For this review, take the finished solid that the model builds, in its own axes (mm). Face numbers are marked on the shaded views. Round coordinates to 2 decimals unless told otherwise and drop trailing zeros. Write each loop counter-clockwise with the first axis right and the second up, starting at its lowest first coordinate (ties: lowest second). Pieces come first, ordered by that corner, then holes. Notation, with made-up numbers: (-28, 29.25) -> (20, 29.25) arc R27 ccw to (20, 60.25) -> close; hole circle Ø7 at (31, 83). An arc over 180 degrees is marked (long way). Answer in a Markdown table with one row per item.
from build123d import *

# Parameters (mm, degrees)
BOSS_EXTRUDE1_DEPTH    = 2.6
BOSS_EXTRUDE2_START    = -2.6
BOSS_EXTRUDE2_DEPTH    = 69
BOSS_EXTRUDE3_START    = 3.2
BOSS_EXTRUDE3_DEPTH    = 2.6
FILL_START             = -63.4
FILL_PATTERN1_DEPTH    = 2.6
FILL_START_2           = -57.9
FILL_PATTERN1_2_DEPTH  = 2.6
FILL_START_3           = -52.4
FILL_PATTERN1_3_DEPTH  = 2.6
FILL_START_4           = -46.9
FILL_PATTERN1_4_DEPTH  = 2.6
FILL_START_5           = -41.4
FILL_PATTERN1_5_DEPTH  = 2.6
FILL_START_6           = -35.9
FILL_PATTERN1_6_DEPTH  = 2.6
FILL_START_7           = -30.4
FILL_PATTERN1_7_DEPTH  = 2.6
FILL_START_8           = -24.9
FILL_PATTERN1_8_DEPTH  = 2.6
FILL_START_9           = -19.4
FILL_PATTERN1_9_DEPTH  = 2.6
FILL_START_10          = -13.9
FILL_PATTERN1_10_DEPTH = 2.6
BOSS_EXTRUDE4_DEPTH    = 14
BOSS_EXTRUDE5_DEPTH    = 1.2
SKETCH6_W              = 9.5
SKETCH6_H              = 1.2
CUT_EXTRUDE1_DEPTH     = 3
CHAMFER1_START         = -1
CHAMFER1_DEPTH         = 3.165267299


with BuildPart() as part:
    # Sketch2 → Boss-Extrude1 (new body)
    with BuildSketch(Plane(origin=(0, 0, 0), x_dir=(0, 0, -1), z_dir=(1, 0, 0))):
        Polygon((0, 0), (0, 5.5), (7.5, 0), align=None)
    boss_extrude1 = extrude(amount=-BOSS_EXTRUDE1_DEPTH)

    # Sketch3 → Boss-Extrude2 (add)
    with BuildSketch(Plane.ZY.offset(2.6).offset(BOSS_EXTRUDE2_START)):
        Polygon((0, 0), (0, 4.879964159), (-6.65449658, 0), align=None)
    extrude(amount=BOSS_EXTRUDE2_DEPTH)

    # Sketch3<3> → Boss-Extrude3 (add)
    with BuildSketch(Plane.ZY.offset(2.6).offset(BOSS_EXTRUDE3_START)):
        Polygon((-6.65449658, 0), (0, 4.879964159), (0, 5.5), (-7.5, 0), align=None)
    extrude(amount=BOSS_EXTRUDE3_DEPTH)

    # Mirror1: Boss-Extrude1 across plane
    add(boss_extrude1.mirror(Plane(origin=(-34.5, 0, 0), x_dir=(0, 0, 1), z_dir=(1, 0, 0))))

    # Fill Pattern1: read off the stored shape, not the designer's step
    # Fill Pattern1 outline → Fill Pattern1 (add)
    with BuildSketch(Plane.YZ.offset(FILL_START)):
        Polygon((4.879964159, 0), (0, -6.65449658), (0, -7.5), (5.5, 0), align=None)
    extrude(amount=FILL_PATTERN1_DEPTH)

    # Fill Pattern1 2 outline → Fill Pattern1 2 (add)
    with BuildSketch(Plane.YZ.offset(FILL_START_2)):
        Polygon((4.879964159, 0), (0, -6.65449658), (0, -7.5), (5.5, 0), align=None)
    extrude(amount=FILL_PATTERN1_2_DEPTH)

    # Fill Pattern1 3 outline → Fill Pattern1 3 (add)
    with BuildSketch(Plane.YZ.offset(FILL_START_3)):
        Polygon((4.879964159, 0), (0, -6.65449658), (0, -7.5), (5.5, 0), align=None)
    extrude(amount=FILL_PATTERN1_3_DEPTH)

    # Fill Pattern1 4 outline → Fill Pattern1 4 (add)
    with BuildSketch(Plane.YZ.offset(FILL_START_4)):
        Polygon((4.879964159, 0), (0, -6.65449658), (0, -7.5), (5.5, 0), align=None)
    extrude(amount=FILL_PATTERN1_4_DEPTH)

    # Fill Pattern1 5 outline → Fill Pattern1 5 (add)
    with BuildSketch(Plane.YZ.offset(FILL_START_5)):
        Polygon((4.879964159, 0), (0, -6.65449658), (0, -7.5), (5.5, 0), align=None)
    extrude(amount=FILL_PATTERN1_5_DEPTH)

    # Fill Pattern1 6 outline → Fill Pattern1 6 (add)
    with BuildSketch(Plane.YZ.offset(FILL_START_6)):
        Polygon((4.879964159, 0), (0, -6.65449658), (0, -7.5), (5.5, 0), align=None)
    extrude(amount=FILL_PATTERN1_6_DEPTH)

    # Fill Pattern1 7 outline → Fill Pattern1 7 (add)
    with BuildSketch(Plane.YZ.offset(FILL_START_7)):
        Polygon((4.879964159, 0), (0, -6.65449658), (0, -7.5), (5.5, 0), align=None)
    extrude(amount=FILL_PATTERN1_7_DEPTH)

    # Fill Pattern1 8 outline → Fill Pattern1 8 (add)
    with BuildSketch(Plane.YZ.offset(FILL_START_8)):
        Polygon((4.879964159, 0), (0, -6.65449658), (0, -7.5), (5.5, 0), align=None)
    extrude(amount=FILL_PATTERN1_8_DEPTH)

    # Fill Pattern1 9 outline → Fill Pattern1 9 (add)
    with BuildSketch(Plane.YZ.offset(FILL_START_9)):
        Polygon((4.879964159, 0), (0, -6.65449658), (0, -7.5), (5.5, 0), align=None)
    extrude(amount=FILL_PATTERN1_9_DEPTH)

    # Fill Pattern1 10 outline → Fill Pattern1 10 (add)
    with BuildSketch(Plane.YZ.offset(FILL_START_10)):
        Polygon((4.879964159, 0), (0, -6.65449658), (0, -7.5), (5.5, 0), align=None)
    extrude(amount=FILL_PATTERN1_10_DEPTH)

    # Sketch4 → Boss-Extrude4 (add)
    with BuildSketch(Plane.ZY.offset(69)):
        with BuildLine():
            Line((0, 2.406191741), (0, 4.879964159))
            Line((0, 4.879964159), (-3.932237623, 1.996323235))
            ThreePointArc((-3.932237623, 1.996323235), (-1.977221876, 2.307779179), (0, 2.406191741))
        make_face()
        with BuildLine():
            Line((0, 4.879964159), (0, 5.5))
            Line((0, 5.5), (-5.225299515, 1.668113689))
            ThreePointArc((-5.225299515, 1.668113689), (-4.581760916, 1.844007543), (-3.932237623, 1.996323235))
            Line((-3.932237623, 1.996323235), (0, 4.879964159))
        make_face()
        with BuildLine():
            Line((-5.225299515, 1.668113689), (0, 5.5))
            Line((0, 5.5), (3.5, 5.5))
            Line((3.5, 5.5), (3.5, 8.5))
            Line((3.5, 8.5), (1.525445934, 8.5))
            Line((1.525445934, 8.5), (-9.5, 2.081639323))
            Line((-9.5, 2.081639323), (-9.5, -0.204677967))
            ThreePointArc((-9.5, -0.204677967), (-7.422606569, 0.868570996), (-5.225299515, 1.668113689))
        make_face()
    boss_extrude4 = extrude(amount=BOSS_EXTRUDE4_DEPTH)

    # Sketch5 → Boss-Extrude5 (add)
    with BuildSketch(Plane.ZY.offset(83)):
        Polygon((3.5, 8.5), (1.525445934, 8.5), (-9.5, 2.081639323), (-9.5, -2.683513675), (3.5, -2.683513675), align=None)
    boss_extrude5 = extrude(amount=-BOSS_EXTRUDE5_DEPTH)

    # Sketch6 → Cut-Extrude1 (cut)
    with BuildSketch(Plane(origin=(0, 8.5, 0), x_dir=(1, 0, 0), z_dir=(0, 1, 0))):
        with Locations((-76.75, -2.9)):
            Rectangle(SKETCH6_W, SKETCH6_H)
    cut_extrude1 = extrude(amount=-CUT_EXTRUDE1_DEPTH, mode=Mode.SUBTRACT)

    # Chamfer1: read off the stored shape, not the designer's step
    # Chamfer1 outline → Chamfer1 (cut)
    with BuildSketch(Plane(origin=(0, 0, 0), x_dir=(1, 0, 0), z_dir=(0, 0.6951264470531402, -0.7188874895331522)).offset(CHAMFER1_START)):
        Polygon((-69, -1.239281183), (-81.8, -1.239281183), (-81.8, -2.239281185), (-69, -2.239281183), align=None)
    chamfer1 = extrude(amount=CHAMFER1_DEPTH, mode=Mode.SUBTRACT)

    # Mirror2: Boss-Extrude4, Boss-Extrude5, Cut-Extrude1, Chamfer1 across plane
    add(boss_extrude4.mirror(Plane(origin=(-34.5, 0, 0), x_dir=(0, 0, 1), z_dir=(1, 0, 0))))
    add(boss_extrude5.mirror(Plane(origin=(-34.5, 0, 0), x_dir=(0, 0, 1), z_dir=(1, 0, 0))))
    add(cut_extrude1.mirror(Plane(origin=(-34.5, 0, 0), x_dir=(0, 0, 1), z_dir=(1, 0, 0))), mode=Mode.SUBTRACT)
    add(chamfer1.mirror(Plane(origin=(-34.5, 0, 0), x_dir=(0, 0, 1), z_dir=(1, 0, 0))), mode=Mode.SUBTRACT)


solid = part.part
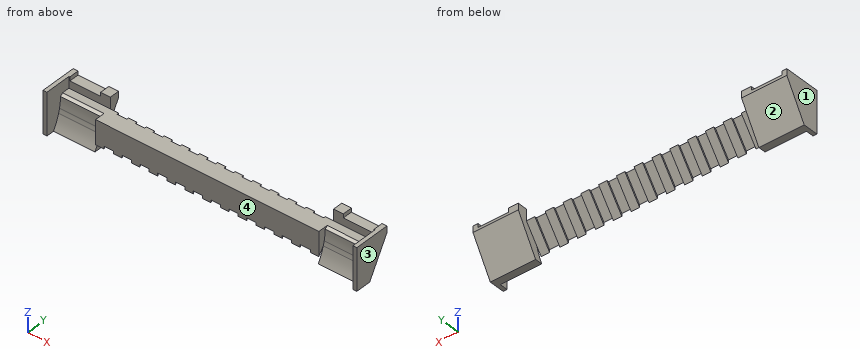
1) For line 1 (X direction, y = 6.5, z = 2.5); line 2 (X direction, y = 4.5, z = 2); line 3 (X direction, y = 3.25, z = -5.5), list the stretches that pass through material, from the lowest coordinate up. Write a range as [from, to].
Solved:
| item | result |
|---|---|
| line 1 | [-83, -81.5], [-72, -69], [0, 3], [12.5, 14] |
| line 2 | [-83, -81.8], [12.8, 14] |
| line 3 | [-83, -69], [0, 14] |
2) Mouldability with a two-part tool opening along X and no side actions: class the marked faces 1, 2, 3 and 4 as pulls with the +X half, pulls with the -X half, needs draft (parallel to the pull), parting line crosses it, or undercut.
Solved:
| item | result |
|---|---|
| face 1 | pulls with the -X half |
| face 2 | needs draft |
| face 3 | pulls with the +X half |
| face 4 | undercut |
3) Clearance check with flat-ended pins moving along their axes: pin 1 Ø4 at (x, z) = (-42.5, -5.5) entering from -Y; pin 2 Ø1.5 at (x, z) = (-8, -5.5) entering from +Y; pin 3 Ø2 at (x, y) = (-22, 3.5) entering from -Z. State where each tip first meets the part, or that it passes through.
Solved:
| item | result |
|---|---|
| pin 1 | y = 0 |
| pin 2 | y = 2.02 |
| pin 3 | z = -4.03 |
4) Consider section A-A on x = -9.5. State the section outline as (y, z) points.
Solved:
| item | result |
|---|---|
| outline | (0, -6.65) -> (4.88, 0) -> (0, 0) -> close |
